Design review of the part shown in the three views and the two pictorial views. Dimensions are in mm from the part's minimum x, y and z. Round coordinates to 2 decimals unless told otherwise and drop trailing zeros. Loops run counter-clockwise (first coordinate to the right, second up) from the corner with the lowest first, then second, coordinate; pieces in that order, holes last. Notation, with made-up numbers: (59.25, -39) - (68.25, -39) arc R38 cw to (68.25, -1) - close; hole circle Ø2 at (40, -29). An arc over 180 degrees is marked (long way). Return JSON: item names as keys, results as strings. Group by question number.
(1) Clearance check with flat-ended pins moving along their axes: pin 1 (6 mm diameter, centred on x = 35.5, z = 7, fed in from -Y); pin 2 (3 mm diameter, centred on y = 4.5, z = 13, fed in from -X); pin 3 (1 mm diameter, centred on y = 4, z = 21, fed in from -X); pin 4 (3 mm diameter, centred on y = 4.5, z = 12, fed in from +X). State where each tip first meets the part, or that it passes through.
(2) We need section A-A, the plane y = 1.55. Write out the cut boundary in (x, z).
(3) We need section C-C, the plane z = 3.81. Write out the cut boundary in (x, y).
(4) We need section B-B, the plane x = 55. Write out the cut boundary in (y, z).
(5) Wall thickness on L1, parallel to Z at x = 72.39, y = 4; L2, parallel to Z at x = 59, y = 4.45; L3, parallel to Y at x = 58, z = 23.25: over which ranges is each line inside the solid? List them lowest first. Write a range as [from, to].
(6) The part is to be moulded in two halves that separate along X. For the marked faces 1 and 2, say which applies: pulls with the +X half, pulls with the -X half, needs draft (parallel to the pull), parting line crosses it, or undercut.
(7) We need section D-D, the plane x = 3.81. Write out the cut boundary in (y, z).
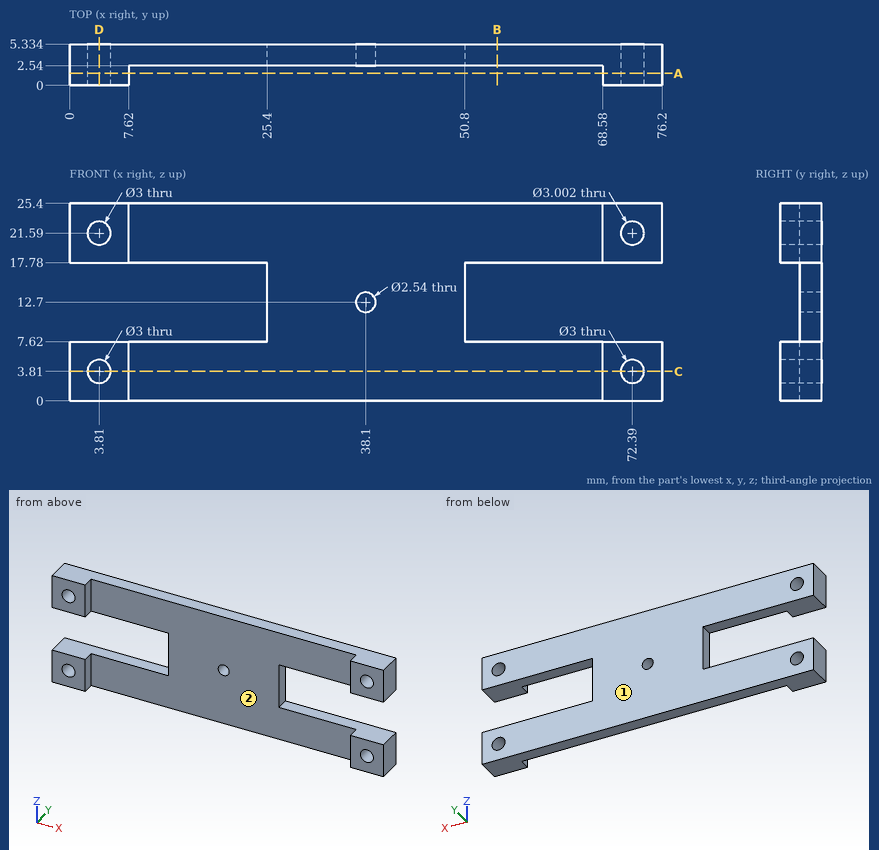
Solutions:
{
 "1": {"pin 1": "y = 2.54", "pin 2": "x = 25.4", "pin 3": "x = 0", "pin 4": "x = 50.8"},
 "2": {"outline": "(0, 0) - (7.62, 0) - (7.62, 7.62) - (0, 7.62) - close; (0, 17.78) - (7.62, 17.78) - (7.62, 25.4) - (0, 25.4) - close; (68.58, 0) - (76.2, 0) - (76.2, 7.62) - (68.58, 7.62) - close; (68.58, 17.78) - (76.2, 17.78) - (76.2, 25.4) - (68.58, 25.4) - close; hole circle Ø3 at (3.81, 3.81); hole circle Ø3 at (3.81, 21.59); hole circle Ø3 at (72.39, 3.81); hole circle Ø3 at (72.39, 21.59)"},
 "3": {"outline": "(0, 0) - (2.31, 0) - (2.31, 5.33) - (0, 5.33) - close; (5.31, 0) - (7.62, 0) - (7.62, 2.54) - (68.58, 2.54) - (68.58, 0) - (70.89, 0) - (70.89, 5.33) - (5.31, 5.33) - close; (73.89, 0) - (76.2, 0) - (76.2, 5.33) - (73.89, 5.33) - close"},
 "4": {"outline": "(2.54, 0) - (5.33, 0) - (5.33, 7.62) - (2.54, 7.62) - close; (2.54, 17.78) - (5.33, 17.78) - (5.33, 25.4) - (2.54, 25.4) - close"},
 "5": {"L1": "[0, 2.31], [5.31, 7.62], [17.78, 20.09], [23.09, 25.4]", "L2": "[0, 7.62], [17.78, 25.4]", "L3": "[2.54, 5.33]"},
 "6": {"face 1": "needs draft", "face 2": "undercut"},
 "7": {"outline": "(0, 0) - (5.33, 0) - (5.33, 2.31) - (0, 2.31) - close; (0, 5.31) - (5.33, 5.31) - (5.33, 7.62) - (0, 7.62) - close; (0, 17.78) - (5.33, 17.78) - (5.33, 20.09) - (0, 20.09) - close; (0, 23.09) - (5.33, 23.09) - (5.33, 25.4) - (0, 25.4) - close"}
}
